Geometry check sheet. Reference: the model listing, model coordinates, mm. A direction names the side the tool comes from. Round coordinates to 2 decimals unless told otherwise and drop trailing zeros. Loops run counter-clockwise (first coordinate to the right, second up) from the corner with the lowest first, then second, coordinate; pieces in that order, holes last. Notation, with made-up numbers: M 35.25,84.25 L 61.25,84.25 A19 cw 61.25,112.25 Z; hole C 75.25,34 d6. An arc over 180 degrees is marked long. Use one line per item in the form item = value. Start each with the question number.
1. Cross-section at B-B (y = -20.2). Record the boundary of the cut face in (x, z).
2. Cross-section at C-C (z = -2). Record the boundary of the cut face in (x, y) (3 decimals), then the cut area to 3 significant figures.
3. Cross-section at A-A (x = 21.06). Record the boundary of the cut face in (y, z).
4. Set-up check for faces 4 (the flat face through (17, -20, 3)), 5 (the flat face through (35, -10.42, 0)), 6 (the flat face through (17, -20, -3)): record each of +Z, -Z, +X, -X, +Y, -Y from which the full face is reachable in a straight line by a thin tool's end or side.
5. Cross-section at D-D (x = 16.5). Record the boundary of the cut face in (y, z).
6. Material ranges on line 1 (Y direction, x = 21.06, z = -0.15); line 2 (Z direction, x = 9, y = -15.5); line 3 (Y direction, x = 5, z = 5.75), recorded low to high.
7. Go/stop test with flat-tipped pins: pin 1 (8 mm diameter, centred on y = -23.5, z = -3.5, fed in from +X); pin 2 (1 mm diameter, centred on x = 12, z = 6.5, fed in from -Y); pin 3 (6 mm diameter, centred on x = 24, y = -15, fed in from +Z). Record where each tip stops, or that it passes through.
8. Draft check along Y on faces 1 (the flat face through (0, -5, 0)), 2 (the flat face through (7, -10.42, 0)), 3 (the flat face through (21, -30, 0)). Enter one of: pulls with the +Y half, pulls with the -Y half, needs draft (parallel to the pull), parting line crosses it, or undercut.
```python
from build123d import *

# Parameters (mm, degrees)
SKETCH1_W           = 42.12
SKETCH1_H           = 10
BOSS_EXTRUDE1_DEPTH = 10
SKETCH2_R           = 2.8
BOSS_EXTRUDE2_DEPTH = 3


with BuildPart() as part:
    # Sketch1 → Boss-Extrude1 (new, symmetric)
    with BuildSketch(Plane.XY):
        with Locations((21.06, -5)):
            Rectangle(SKETCH1_W, SKETCH1_H)
    extrude(amount=BOSS_EXTRUDE1_DEPTH, both=True)

    # Sketch2 → Boss-Extrude2 (add, symmetric)
    with BuildSketch(Plane.XY):
        with BuildLine():
            Line((11.595, -30), (30.525, -30))
            ThreePointArc((30.525, -30), (34.684463962, -20.214378878), (30.545664183, -10.42))
            Line((30.545664183, -10.42), (39.681383671, -10.42))
            Line((39.681383671, -10.42), (39.681383671, -10))
            Line((39.681383671, -10), (2.438616329, -10))
            Line((2.438616329, -10), (2.438616329, -10.42))
            Line((2.438616329, -10.42), (11.574335817, -10.42))
            ThreePointArc((11.574335817, -10.42), (7.435536038, -20.214378878), (11.595, -30))
        make_face()
        with Locations((21.06, -20.2)):
            Circle(SKETCH2_R, mode=Mode.SUBTRACT)
    extrude(amount=BOSS_EXTRUDE2_DEPTH, both=True)


solid = part.part
```
Reported:
q1.outline = M 7.44,-3 L 18.26,-3 L 18.26,3 L 7.44,3 Z; M 23.86,-3 L 34.68,-3 L 34.68,3 L 23.86,3 Z
q2.outline = M 0,-10 L 2.439,-10 L 2.439,-10.42 L 11.574,-10.42 A13.624 ccw 11.595,-30 L 30.525,-30 A13.624 ccw 30.546,-10.42 L 39.681,-10.42 L 39.681,-10 L 42.12,-10 L 42.12,0 L 0,0 Z; hole C 21.06,-20.2 d5.6
q2.area = 895 mm²
q3.outline = M -30,-3 L -23,-3 L -23,3 L -30,3 Z; M -17.4,-3 L -10,-3 L -10,-10 L 0,-10 L 0,10 L -10,10 L -10,3 L -17.4,3 Z
q4.face_4 = +Z, +X, -X, -Y
q4.face_5 = +Z, -Z, +X
q4.face_6 = -Z, +X, -X, -Y
q5.outline = M -30,-3 L -10,-3 L -10,-10 L 0,-10 L 0,10 L -10,10 L -10,3 L -30,3 Z
q6.line_1 = -30 to -23, -17.4 to 0
q6.line_2 = -3 to 3
q6.line_3 = -10 to 0
q7.pin_1 = 34.68
q7.pin_2 = -10
q7.pin_3 = 3
q8.face_1 = needs draft
q8.face_2 = undercut
q8.face_3 = pulls with the -Y half
